Design review of the part built by this model. Coordinates are the model's own, in mm. A direction names the side the tool comes from. Give positions to 0.01 mm unless a question says otherwise; leave off trailing zeros. Write each loop counter-clockwise with the first axis right and the second up, starting at its lowest first coordinate (ties: lowest second). Pieces come first, ordered by that corner, then holes. Notation, with made-up numbers: M 63,43.25 L 103,43.25 A31 cw 103,75.25 Z; hole C 69,-19 d2. An arc over 180 degrees is marked long. Answer in a Markdown table with one row per item.
```python
from build123d import *

# Parameters (mm, degrees)
F0_R     = 10
F1_DEPTH = 15


with BuildPart() as f1:
    # F0 (on Top) → F1 (new body)
    with BuildSketch(Plane.XY):
        with BuildLine():
            Line((76, 78.5), (-76, 78.5))
            ThreePointArc((-76, 78.5), (-79.535534, 77.035534), (-81, 73.5))
            Line((-81, 73.5), (-81, -73.5))
            ThreePointArc((-81, -73.5), (-79.535534, -77.035534), (-76, -78.5))
            Line((-76, -78.5), (76, -78.5))
            ThreePointArc((76, -78.5), (79.535534, -77.035534), (81, -73.5))
            Line((81, -73.5), (81, 73.5))
            ThreePointArc((81, 73.5), (79.535534, 77.035534), (76, 78.5))
        make_face()
        with BuildLine():
            ThreePointArc((-61, 57.5), (-53.5, 65), (-46, 57.5))
            Line((-46, 57.5), (-46, 0))
            Line((-46, 0), (-46, -57.5))
            ThreePointArc((-46, -57.5), (-53.5, -65), (-61, -57.5))
            Line((-61, -57.5), (-61, 0))
            Line((-61, 0), (-61, 57.5))
        make_face(mode=Mode.SUBTRACT)
        Circle(F0_R, mode=Mode.SUBTRACT)
        with BuildLine():
            Line((46, 0), (46, 57.5))
            ThreePointArc((46, 57.5), (53.5, 65), (61, 57.5))
            Line((61, 57.5), (61, 0))
            Line((61, 0), (61, -57.5))
            ThreePointArc((61, -57.5), (53.5, -65), (46, -57.5))
            Line((46, -57.5), (46, 0))
        make_face(mode=Mode.SUBTRACT)
    extrude(amount=F1_DEPTH)


solid = f1.part
```
1) Add section B-B (y = 0). Write out the cut boundary in (x, z).
Geometry says:
| item | result |
|---|---|
| outline | M -81,0 L -61,0 L -61,15 L -81,15 Z; M -46,0 L -10,0 L -10,15 L -46,15 Z; M 10,0 L 46,0 L 46,15 L 10,15 Z; M 61,0 L 81,0 L 81,15 L 61,15 Z |
2) Add section A-A (x = 0). Write out the cut boundary in (y, z), and give its area (4 significant figures).
Geometry says:
| item | result |
|---|---|
| outline | M -78.5,0 L -10,0 L -10,15 L -78.5,15 Z; M 10,0 L 78.5,0 L 78.5,15 L 10,15 Z |
| area | 2,055 mm^2 |
3) For faces 4 (the face through (1, 78.5, 7)), 5 (the face through (-61, -1, 7)), list the 3-axis set-ups (+Z, -Z, +X, -X, +Y, -Y) from which the entire face can be reached by the end or side of a thin tool; tool diameter is ignored.
Geometry says:
| item | result |
|---|---|
| face 4 | +Z, -Z, +X, -X, +Y |
| face 5 | +Z, -Z |
4) To check wall thickness, follow probe 1 along Y at (x, z) = (0, 4.5); probe 2 along X at (y, z) = (22, 13.5); probe 3 along Y at (x, z) = (5.5, 1.25). State the ranges of each line that lie inside material, in increasing order. Write a range as [from, to].
Geometry says:
| item | result |
|---|---|
| probe 1 | [-78.5, -10], [10, 78.5] |
| probe 2 | [-81, -61], [-46, 46], [61, 81] |
| probe 3 | [-78.5, -8.35], [8.35, 78.5] |
5) The part is to be moulded in two halves that separate along Y. For faces 1 (the face through (-1, 19, 0)), 2 (the face through (53.66, -65, 7.4)), 3 (the face through (-1, -78.5, 7)), say which applies: released by +Y, released by -Y, zero draft, split by the parting line, or undercut.
Geometry says:
| item | result |
|---|---|
| face 1 | zero draft |
| face 2 | undercut |
| face 3 | released by -Y |
6) Add section D-D (y = 43). Write out the cut boundary in (x, z), and give its area (3 significant figures).
Geometry says:
| item | result |
|---|---|
| outline | M -81,0 L -61,0 L -61,15 L -81,15 Z; M -46,0 L 46,0 L 46,15 L -46,15 Z; M 61,0 L 81,0 L 81,15 L 61,15 Z |
| area | 1,980 mm^2 |
7) Add section C-C (z = 8). Write out the cut boundary in (x, y), and give its area (3 significant figures).
Geometry says:
| item | result |
|---|---|
| outline | M -81,-73.5 A5 ccw -76,-78.5 L 76,-78.5 A5 ccw 81,-73.5 L 81,73.5 A5 ccw 76,78.5 L -76,78.5 A5 ccw -81,73.5 Z; hole M -61,-57.5 A7.5 ccw -46,-57.5 L -46,57.5 A7.5 ccw -61,57.5 Z; hole C 0,0 d20; hole M 46,-57.5 A7.5 ccw 61,-57.5 L 61,57.5 A7.5 ccw 46,57.5 Z |
| area | 21,300 mm^2 |
